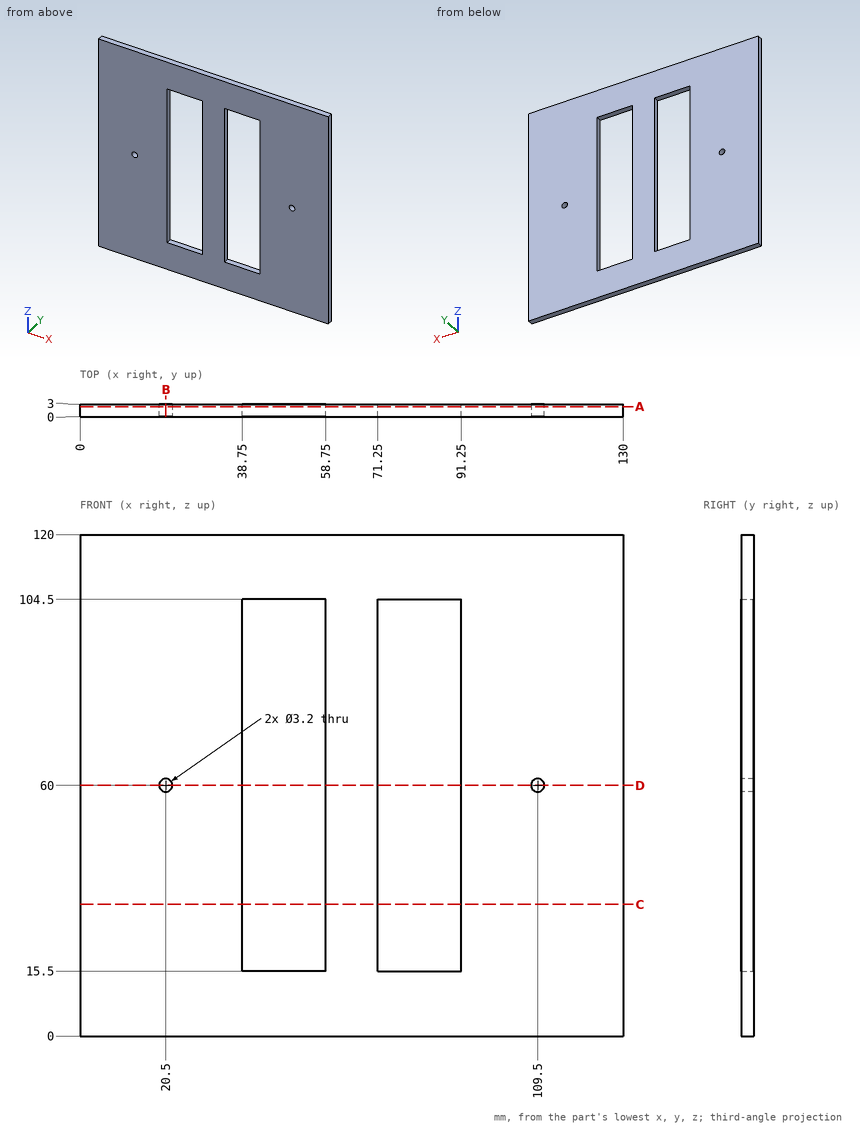
Verification items for this drawing (mm, ordinates from the low corner). Give positions to 0.01 mm unless a question says otherwise; leave off trailing zeros. Write each loop counter-clockwise with the first axis right and the second up, starting at its lowest first coordinate (ties: lowest second). Pieces come first, ordered by that corner, then holes. Notation, with made-up numbers: (-12, 68) -> (16, 68) arc R12 ccw to (16, 77) -> close; hole circle Ø3 at (-4, -35). An arc over 180 degrees is marked (long way). Write item = value, one per line.
Item 1: Gauge pin test, flat ends, axial feed: pin 1 (1.5 mm diameter, centred on x = 53.5, y = 1.5, fed in from -Z); pin 2 (2.5 mm diameter, centred on x = 20.5, z = 60, fed in from +Y). Record the tip position at first contact, or that the pin passes through.
Output:
pin_1 = 0
pin_2 = through
Item 2: Sectioned sample at D-D on z = 60. Record the boundary of the cut face in (x, y).
Output:
outline = (0, 0) -> (18.9, 0) -> (18.9, 3) -> (0, 3) -> close; (22.1, 0) -> (38.75, 0) -> (38.75, 3) -> (22.1, 3) -> close; (58.75, 0) -> (71.25, 0) -> (71.25, 3) -> (58.75, 3) -> close; (91.25, 0) -> (107.9, 0) -> (107.9, 3) -> (91.25, 3) -> close; (111.1, 0) -> (130, 0) -> (130, 3) -> (111.1, 3) -> close
Item 3: Sectioned sample at A-A on y = 2.4. Record the boundary of the cut face in (x, z).
Output:
outline = (0, 0) -> (130, 0) -> (130, 120) -> (0, 120) -> close; hole circle Ø3.2 at (20.5, 60); hole (38.75, 15.5) -> (58.75, 15.5) -> (58.75, 104.5) -> (38.75, 104.5) -> close; hole (71.25, 15.5) -> (91.25, 15.5) -> (91.25, 104.5) -> (71.25, 104.5) -> close; hole circle Ø3.2 at (109.5, 60)
Item 4: Scan lines: probe 1 along X at (y, z) = (0.9, 80.5); probe 2 along Z at (x, y) = (109.5, 1.35); probe 3 along Z at (x, y) = (89, 1.7). Record each from-to range of solid material in increasing order. Write a range as from..to.
Output:
probe_1 = 0..38.75, 58.75..71.25, 91.25..130
probe_2 = 0..58.4, 61.6..120
probe_3 = 0..15.5, 104.5..120
Item 5: Sectioned sample at B-B on x = 20.5. Record the boundary of the cut face in (y, z), and give its area (3 significant figures).
Output:
outline = (0, 0) -> (3, 0) -> (3, 58.4) -> (0, 58.4) -> close; (0, 61.6) -> (3, 61.6) -> (3, 120) -> (0, 120) -> close
area = 350 mm^2
Item 6: Sectioned sample at C-C on z = 31.5. Record the boundary of the cut face in (x, y), and give its area (3 significant figures).
Output:
outline = (0, 0) -> (38.75, 0) -> (38.75, 3) -> (0, 3) -> close; (58.75, 0) -> (71.25, 0) -> (71.25, 3) -> (58.75, 3) -> close; (91.25, 0) -> (130, 0) -> (130, 3) -> (91.25, 3) -> close
area = 270 mm^2
